Geometry check sheet. Reference: the model listing, model coordinates, mm. Face numbers are marked on the shaded views. A direction names the side the tool comes from. Give positions to 0.01 mm unless a question says otherwise; leave off trailing zeros. Loops run counter-clockwise (first coordinate to the right, second up) from the corner with the lowest first, then second, coordinate; pieces in that order, holes last. Notation, with made-up numbers: (35.25, 22.25) - (61.25, 22.25) arc R11 ccw to (61.25, 38.25) - close; hole circle Ø10 at (67, 39). An arc over 180 degrees is marked (long way). One line per question, with ' | ' between items. Start each with the question number.
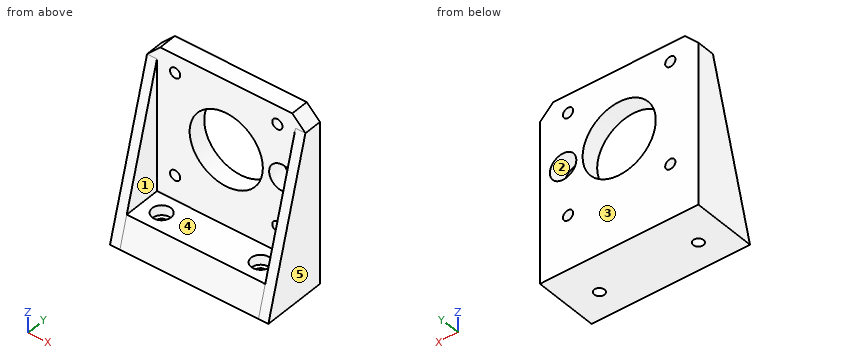
from build123d import *

# Parameters (mm, degrees)
CROQUIS1_R                 = 1.55
CROQUIS1_R_2               = 11.1
CROQUIS1_R_3               = 4
SALIENTE_EXTRUIR1_DEPTH    = 5.5
SALIENTE_EXTRUIR2_DEPTH    = 5.5
SALIENTE_EXTRUIR3_DEPTH    = 3
SALIENTE_EXTRUIR4_DEPTH    = 5.5
SALIENTE_EXTRUIR5_DEPTH    = 3
CROQUIS7_W                 = 42
CROQUIS7_H                 = 9
SALIENTE_EXTRUIR6_DEPTH    = 14
CROQUIS9_R                 = 1.55
CORTAR_EXTRUIR1_DEPTH      = 9
CROQUIS10_R                = 2.85
CROQUIS10_R_2              = 1.55
CORTAR_EXTRUIR2_DEPTH      = 3
CORTAR_EXTRUIR3_DEPTH      = 4
CORTAR_EXTRUIR3_DEPTH_BACK = 46


with BuildPart() as part:
    # Croquis1 → Saliente-Extruir1 (new body)
    with BuildSketch(Plane(origin=(0, 0, 0), x_dir=(1, 0, 0), z_dir=(0, 1, 0))):
        Polygon((0, 4), (0, 49), (4, 53), (44, 53), (48, 49), (48, 4), (44, 0), (4, 0), align=None)
        with Locations((8.5, 36.5)):
            Circle(CROQUIS1_R, mode=Mode.SUBTRACT)
        with Locations((39.5, 36.5)):
            Circle(CROQUIS1_R, mode=Mode.SUBTRACT)
        with Locations((8.5, 5.5)):
            Circle(CROQUIS1_R, mode=Mode.SUBTRACT)
        with Locations((39.5, 5.5)):
            Circle(CROQUIS1_R, mode=Mode.SUBTRACT)
        with Locations((24, 21)):
            Circle(CROQUIS1_R_2, mode=Mode.SUBTRACT)
        with Locations((41, 21)):
            Circle(CROQUIS1_R_3, mode=Mode.SUBTRACT)
    extrude(amount=SALIENTE_EXTRUIR1_DEPTH)

    # Croquis3 → Saliente-Extruir2 (add)
    with BuildSketch(Plane(origin=(0, 5.5, 0), x_dir=(1, 0, 0), z_dir=(0, 1, 0))):
        Polygon((4, 53), (0, 53), (0, 49), align=None)
    extrude(amount=-SALIENTE_EXTRUIR2_DEPTH)

    # Croquis4 → Saliente-Extruir3 (add)
    with BuildSketch(Plane.ZY):
        Polygon((-53, 0), (-53, 5.5), (-4, 5.5), (-4, 0), (-53, -14), align=None)
    extrude(amount=-SALIENTE_EXTRUIR3_DEPTH)

    # Croquis5 → Saliente-Extruir4 (add)
    with BuildSketch(Plane(origin=(0, 5.5, 0), x_dir=(1, 0, 0), z_dir=(0, 1, 0))):
        Polygon((48, 49), (48, 53), (44, 53), align=None)
    extrude(amount=-SALIENTE_EXTRUIR4_DEPTH)

    # Croquis6 → Saliente-Extruir5 (add)
    with BuildSketch(Plane(origin=(48, 0, 0), x_dir=(0, 0, -1), z_dir=(1, 0, 0))):
        Polygon((4, 5.5), (4, 0), (53, -14), (53, 0), (53, 5.5), align=None)
    extrude(amount=-SALIENTE_EXTRUIR5_DEPTH)

    # Croquis7 → Saliente-Extruir6 (add)
    with BuildSketch(Plane.XZ):
        with Locations((24, -48.5)):
            Rectangle(CROQUIS7_W, CROQUIS7_H)
    extrude(amount=SALIENTE_EXTRUIR6_DEPTH)

    # Croquis9 → Cortar-Extruir1 (cut)
    with BuildSketch(Plane.XY.offset(-44)):
        with Locations((9, -5.714285714)):
            Circle(CROQUIS9_R)
        with Locations((39, -5.714285714)):
            Circle(CROQUIS9_R)
    extrude(amount=-CORTAR_EXTRUIR1_DEPTH, mode=Mode.SUBTRACT)

    # Croquis10 → Cortar-Extruir2 (cut)
    with BuildSketch(Plane.XY.offset(-44)):
        with Locations((9, -5.714285714)):
            Circle(CROQUIS10_R)
        with Locations((9, -5.714285714)):
            Circle(CROQUIS10_R_2, mode=Mode.SUBTRACT)
        with Locations((39, -5.714285714)):
            Circle(CROQUIS10_R)
        with Locations((39, -5.714285714)):
            Circle(CROQUIS10_R_2, mode=Mode.SUBTRACT)
    extrude(amount=-CORTAR_EXTRUIR2_DEPTH, mode=Mode.SUBTRACT)

    # Croquis11 → Cortar-Extruir3 (cut, two sides)
    with BuildSketch(Plane.ZY.offset(-3)) as cortar_extruir3_sk:
        Polygon((-44, -11.428571429), (-53, -14), (-44, -14), align=None)
    extrude(amount=CORTAR_EXTRUIR3_DEPTH, mode=Mode.SUBTRACT)
    extrude(cortar_extruir3_sk.sketch, amount=-CORTAR_EXTRUIR3_DEPTH_BACK, mode=Mode.SUBTRACT)


solid = part.part
(1) Mould release check, pull along X, two halves, no side actions. Record for the marked faces 3, 4 and 5: pulls with the +X half, pulls with the -X half, needs draft (parallel to the pull), parting line crosses it, or undercut.
(2) Section check A-A, the plane x = 24. Record the boundary of the cut face in (y, z).
(3) Section check D-D, the plane x = 39.5. Record the boundary of the cut face in (y, z).
(4) Depth check by flat-ended pin: pin 1 Ø10 at (x, y) = (11.5, -6) entering from +Z; pin 2 Ø10 at (x, z) = (22.5, -23) entering from +Y; pin 3 Ø4 at (x, z) = (39.5, -5.5) entering from -Y; pin 4 Ø3.5 at (x, y) = (39, -5.71) entering from +Z. Enter the tip coordinate at first touch or a pass-through.
(5) Section check C-C, the plane z = -23.5. Record the boundary of the cut face in (x, y).
(6) Section check B-B, the plane y = 4. Record the boundary of the cut face in (x, z), and give its area (3 significant figures).
(7) Tool access check on the marked faces 1 and 2. Record the directions out of +Z, -Z, +X, -X, +Y, -Y that give a thin tool (end or side, any length) a straight path to the whole face; none if there is none.
(8) Material ranges on line 1 (X direction, y = 1.1, z = -21); line 2 (Z direction, x = 8.5, y = 2.15); line 3 (Z direction, x = 39.5, y = 2.65), recorded low to high.
Numbers:
1) face 3: needs draft | face 4: undercut | face 5: pulls with the +X half
2) outline: (-14, -53) - (5.5, -53) - (5.5, -32.1) - (0, -32.1) - (0, -44) - (-11.43, -44) - close; (0, -9.9) - (5.5, -9.9) - (5.5, 0) - (0, 0) - close
3) outline: (-14, -53) - (-7.18, -53) - (-7.18, -47) - (-8.52, -47) - (-8.52, -44) - (-11.43, -44) - close; (-4.25, -53) - (5.5, -53) - (5.5, -38.05) - (0, -38.05) - (0, -44) - (-2.91, -44) - (-2.91, -47) - (-4.25, -47) - close; (0, -34.95) - (5.5, -34.95) - (5.5, -24.71) - (0, -24.71) - close; (0, -17.29) - (5.5, -17.29) - (5.5, -7.05) - (0, -7.05) - close; (0, -3.95) - (5.5, -3.95) - (5.5, 0) - (0, 0) - close
4) pin 1: z = -44 | pin 2: through | pin 3: y = 0 | pin 4: z = -47
5) outline: (0, -5.57) - (3, -5.57) - (3, 0) - (13.19, 0) - (13.19, 5.5) - (0, 5.5) - close; (34.81, 0) - (37.88, 0) - (37.88, 5.5) - (34.81, 5.5) - close; (44.12, 0) - (45, 0) - (45, -5.57) - (48, -5.57) - (48, 5.5) - (44.12, 5.5) - close
6) outline: (0, -53) - (48, -53) - (48, -4) - (44, 0) - (4, 0) - (0, -4) - close; hole circle Ø3.1 at (8.5, -36.5); hole circle Ø3.1 at (8.5, -5.5); hole circle Ø22.2 at (24, -21); hole circle Ø8 at (41, -21); hole circle Ø3.1 at (39.5, -36.5); hole circle Ø3.1 at (39.5, -5.5) | area: 2,060 mm^2
7) face 1: +Z, -Y | face 2: +Y, -Y
8) line 1: 0 to 12.9, 35.1 to 37, 45 to 48 | line 2: -53 to -38.05, -34.95 to -7.05, -3.95 to 0 | line 3: -53 to -38.05, -34.95 to -24.71, -17.29 to -7.05, -3.95 to 0
